Study the drawing (mm; zero at the part's minimum x, y, z) and answer. Coordinates: 2 decimals unless noted, no trailing zeros. Loops run counter-clockwise (first coordinate to the right, second up) from the corner with the lowest first, then second, coordinate; pieces in that order, holes last. Notation, with made-up numbers: (39.25, -33.5) - (90.25, -33.5) arc R9 ccw to (90.25, -23.5) - close; hole circle Ø2 at (31.5, -22.5). An arc over 180 degrees is marked (long way). One line per item, written item: value. Start each with the question number.
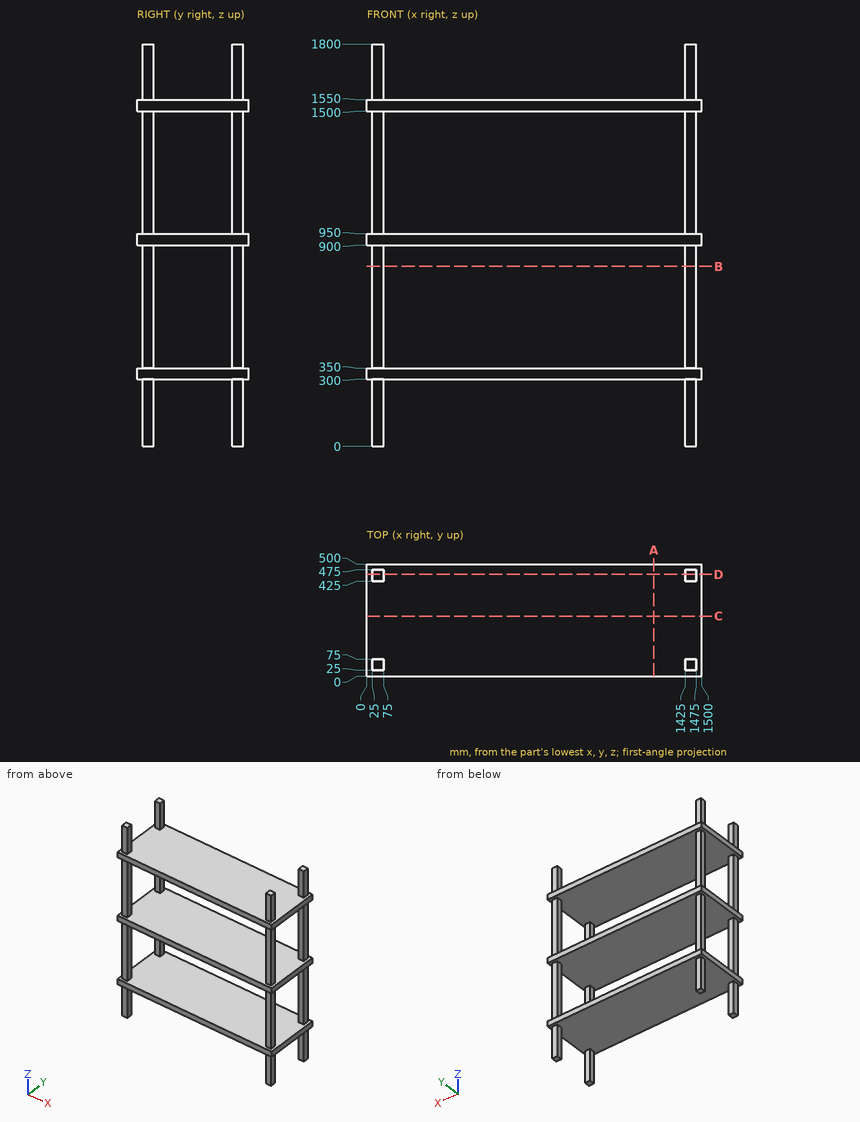
1) Section B-B, the plane z = 805 is taken. Determine the outline of the cut face in (x, y).
2) Section A-A, the plane x = 1285 is taken. Determine the outline of the cut face in (y, z), and give its area (3 significant figures).
3) Section C-C, the plane y = 268 is taken. Determine the outline of the cut face in (x, z).
4) Flat-ended cylindrical pins translate along their axes: P1, Ø10, axis at x = 889, y = 264.5, coming from the -Z side; P2, Ø15, axis at y = 462, z = 591, coming from the +X side; P3, Ø25, axis at y = 51, z = 1670.5, coming from the -X side. Find the tip coordinate at first contact, or state that the pin passes through.
5) Straight lines are drawn through the part: L1, parallel to Z at x = 851, y = 120; L2, parallel to X at y = 70, z = 139. For each, find the intervals that lie inside material, in ascending order.
6) Section D-D, the plane y = 454.5 is taken. State how many separate pieces and enclosed holes the cut face has, and give its area (3 significant figures).
Answer below:
1. outline: (25, 25) - (75, 25) - (75, 75) - (25, 75) - close; (25, 425) - (75, 425) - (75, 475) - (25, 475) - close; (1425, 25) - (1475, 25) - (1475, 75) - (1425, 75) - close; (1425, 425) - (1475, 425) - (1475, 475) - (1425, 475) - close
2. outline: (0, 300) - (500, 300) - (500, 350) - (0, 350) - close; (0, 900) - (500, 900) - (500, 950) - (0, 950) - close; (0, 1500) - (500, 1500) - (500, 1550) - (0, 1550) - close
2. area: 75,000 mm2
3. outline: (0, 300) - (1500, 300) - (1500, 350) - (0, 350) - close; (0, 900) - (1500, 900) - (1500, 950) - (0, 950) - close; (0, 1500) - (1500, 1500) - (1500, 1550) - (0, 1550) - close
4. P1: z = 300
4. P2: x = 1475
4. P3: x = 25
5. L1: 300 to 350, 900 to 950, 1500 to 1550
5. L2: 25 to 75, 1425 to 1475
6. separate pieces: 1
6. enclosed holes: 2
6. area: 390,000 mm2
